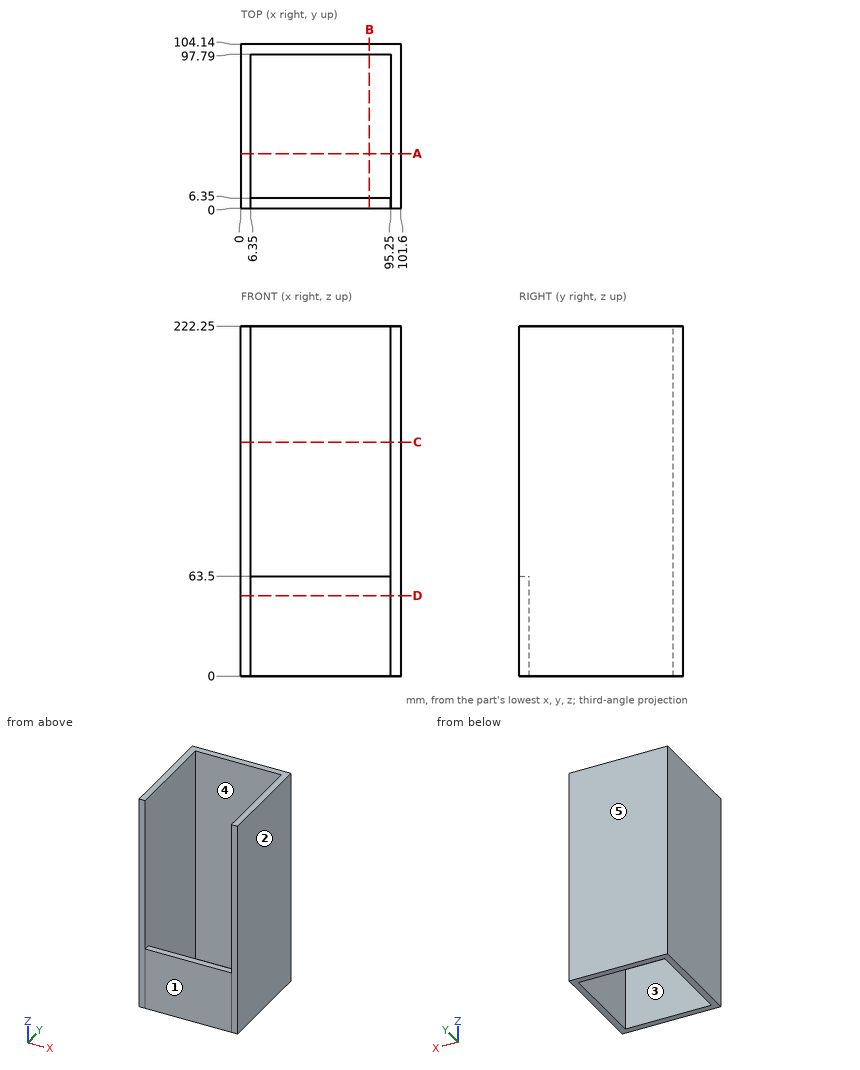
For this review, use the dimensioned drawing (mm, ordinates from the lowest corner) and the shaded views. A direction names the side the tool comes from. Give positions to 0.01 mm unless a question says otherwise; leave off trailing zeros. Write each loop counter-clockwise with the first axis right and the second up, starting at its lowest first coordinate (ties: lowest second). Pieces come first, ordered by that corner, then holes. Notation, with made-up numbers: M 10.25,0 L 68.25,0 A25 ccw 68.25,17 Z; hole C -6,57.5 d10. An arc over 180 degrees is marked long. Answer as a JSON object with one key per item and string values. Group by question number.
Item 1: Consider section D-D on z = 51. Write out the cut boundary in (x, y), plus the area to 3 significant figures.
Item 2: Tool access review of the marked faces 4 and 5: name each direction out of +Z, -Z, +X, -X, +Y, -Y from which nothing blocks a thin tool from reaching the whole face with its end or side.
Item 3: Consider section A-A on y = 34.5. Write out the cut boundary in (x, z), plus the area to 3 significant figures.
Item 4: Consider section C-C on z = 148.5. Write out the cut boundary in (x, y).
Item 5: For pin 1 Ø7 at (x, y) = (71, 3.5) entering from +Z; pin 2 Ø3 at (x, z) = (71.5, 165) entering from -Y, all flat-tipped, find the tip position at first contact; note any pin that passes through.
Item 6: Draft analysis for pull direction X (two halves, no side actions). For the marked faces 1, 2 and 3, state which applies: +X half, -X half, draft (parallel to the pull), parting line (faces both ways), or undercut.
Item 7: Consider section B-B on x = 81.5. Write out the cut boundary in (y, z), plus the area to 3 significant figures.
Item 8: For probe 1 along Y at (x, z) = (88.5, 36); probe 2 along X at (y, z) = (36.5, 94); probe 3 along Y at (x, z) = (50, 172), list the stretches that pass through material, from the lowest coordinate up. Write a range as [from, to].
Check result:
{
 "1": {"outline": "M 0,0 L 101.6,0 L 101.6,104.14 L 0,104.14 Z; hole M 6.35,6.35 L 95.25,6.35 L 95.25,97.79 L 6.35,97.79 Z", "area": "2,450 mm^2"},
 "2": {"face 4": "+Z, -Z", "face 5": "+Z, -Z, +X, -X, +Y"},
 "3": {"outline": "M 0,0 L 6.35,0 L 6.35,222.25 L 0,222.25 Z; M 95.25,0 L 101.6,0 L 101.6,222.25 L 95.25,222.25 Z", "area": "2,820 mm^2"},
 "4": {"outline": "M 0,0 L 6.35,0 L 6.35,97.79 L 95.25,97.79 L 95.25,0 L 101.6,0 L 101.6,104.14 L 0,104.14 Z"},
 "5": {"pin 1": "stops at z = 63.5", "pin 2": "stops at y = 97.79"},
 "6": {"face 1": "draft", "face 2": "+X half", "face 3": "undercut"},
 "7": {"outline": "M 0,0 L 6.35,0 L 6.35,63.5 L 0,63.5 Z; M 97.79,0 L 104.14,0 L 104.14,222.25 L 97.79,222.25 Z", "area": "1,810 mm^2"},
 "8": {"probe 1": "y = [0, 6.35], [97.79, 104.14]", "probe 2": "x = [0, 6.35], [95.25, 101.6]", "probe 3": "y = [97.79, 104.14]"}
}
